Read the model definition and answer for the solid it produces. Units are mm, in the model's axes. A direction names the side the tool comes from. Give positions to 0.01 mm unless a question says otherwise; leave off trailing zeros. Write each loop counter-clockwise with the first axis right and the second up, starting at its lowest first coordinate (ties: lowest second). Pieces come first, ordered by that corner, then holes. Notation, with made-up numbers: (65.5, -40) -> (91.5, -40) arc R26 ccw to (91.5, -5) -> close; hole circle Ø2 at (87.25, 67). An arc over 180 degrees is marked (long way). Write item = value, one per line.
from build123d import *

# Parameters (mm, degrees)
BOSS_EXTRUDE1_DEPTH = 30
SKETCH2_R           = 5
CUT_EXTRUDE1_DEPTH  = 6
SKETCH3_R           = 40
BOSS_EXTRUDE2_DEPTH = 6


with BuildPart() as part:
    # Sketch1 → Boss-Extrude1 (new body)
    with BuildSketch(Plane.XY):
        with BuildLine():
            Line((-2.9, 13.696349879), (-2.9, 16.8))
            Line((-2.9, 16.8), (2.9, 16.8))
            Line((2.9, 16.8), (2.9, 13.696349879))
            ThreePointArc((2.9, 13.696349879), (5.357568053, 12.934313455), (7.634172211, 11.735391542))
            Line((7.634172211, 11.735391542), (9.828784258, 13.930003589))
            Line((9.828784258, 13.930003589), (13.930003589, 9.828784258))
            Line((13.930003589, 9.828784258), (11.735391542, 7.634172211))
            ThreePointArc((11.735391542, 7.634172211), (12.934313455, 5.357568053), (13.696349879, 2.9))
            Line((13.696349879, 2.9), (16.8, 2.9))
            Line((16.8, 2.9), (16.8, -2.9))
            Line((16.8, -2.9), (13.696349879, -2.9))
            ThreePointArc((13.696349879, -2.9), (12.934313455, -5.357568053), (11.735391542, -7.634172211))
            Line((11.735391542, -7.634172211), (13.930003589, -9.828784258))
            Line((13.930003589, -9.828784258), (9.828784258, -13.930003589))
            Line((9.828784258, -13.930003589), (7.634172211, -11.735391542))
            ThreePointArc((7.634172211, -11.735391542), (5.357568053, -12.934313455), (2.9, -13.696349879))
            Line((2.9, -13.696349879), (2.9, -16.8))
            Line((2.9, -16.8), (-2.9, -16.8))
            Line((-2.9, -16.8), (-2.9, -13.696349879))
            ThreePointArc((-2.9, -13.696349879), (-5.357568053, -12.934313455), (-7.634172211, -11.735391542))
            Line((-7.634172211, -11.735391542), (-9.828784258, -13.930003589))
            Line((-9.828784258, -13.930003589), (-13.930003589, -9.828784258))
            Line((-13.930003589, -9.828784258), (-11.735391542, -7.634172211))
            ThreePointArc((-11.735391542, -7.634172211), (-12.934313455, -5.357568053), (-13.696349879, -2.9))
            Line((-13.696349879, -2.9), (-16.8, -2.9))
            Line((-16.8, -2.9), (-16.8, 2.9))
            Line((-16.8, 2.9), (-13.696349879, 2.9))
            ThreePointArc((-13.696349879, 2.9), (-12.934313455, 5.357568053), (-11.735391542, 7.634172211))
            Line((-11.735391542, 7.634172211), (-13.930003589, 9.828784258))
            Line((-13.930003589, 9.828784258), (-9.828784258, 13.930003589))
            Line((-9.828784258, 13.930003589), (-7.634172211, 11.735391542))
            ThreePointArc((-7.634172211, 11.735391542), (-5.357568053, 12.934313455), (-2.9, 13.696349879))
        make_face()
    extrude(amount=BOSS_EXTRUDE1_DEPTH)

    # Sketch2 → Cut-Extrude1 (cut)
    with BuildSketch(Plane(origin=(0, 0, 0), x_dir=(-1, 0, 0), z_dir=(0, 0, -1))):
        Circle(SKETCH2_R)
    extrude(amount=-CUT_EXTRUDE1_DEPTH, mode=Mode.SUBTRACT)

    # Sketch3 → Boss-Extrude2 (add)
    with BuildSketch(Plane.XY.offset(30)):
        Circle(SKETCH3_R)
    extrude(amount=BOSS_EXTRUDE2_DEPTH)


solid = part.part
(1) The part is cut by section B-B on y = 0. Determine the outline of the cut face in (x, z), plus the area to 3 significant figures.
Checks:
outline = (-40, 30) -> (-16.8, 30) -> (-16.8, 0) -> (-5, 0) -> (-5, 6) -> (5, 6) -> (5, 0) -> (16.8, 0) -> (16.8, 30) -> (40, 30) -> (40, 36) -> (-40, 36) -> close
area = 1,430 mm²
(2) A tool of negligible diameter and unlimited length cuts with its end or side. For faces 1 (the cylindrical face through (-5.39, 12.92, 14.79)), 2 (the flat face through (8.7, -12.8, 14.8)), 3 (the flat face through (-12.8, 8.7, 14.8)), 4 (the flat face through (12.8, 8.7, 14.8)), from which of +Z, -Z, +X, -X, +Y, -Y can it reach the whole face along a straight path? Write none if from no direction.
Checks:
face_1 = -Z, +Y
face_2 = -Z, -Y
face_3 = -Z, -X
face_4 = -Z, +X
(3) Consider L1, parallel to Y at x = 0, z = 4.2; L2, parallel to Z at x = -10, y = -16; L3, parallel to X at y = -16, z = 21.5. Determine where each line is inside the solid, lowest interval first.
Checks:
L1 = -16.8 to -5, 5 to 16.8
L2 = 30 to 36
L3 = -2.9 to 2.9
(4) The part is cut by section D-D on y = -15. Determine the outline of the cut face in (x, z), plus the area to 3 significant figures.
Checks:
outline = (-37.08, 30) -> (-2.9, 30) -> (-2.9, 0) -> (2.9, 0) -> (2.9, 30) -> (37.08, 30) -> (37.08, 36) -> (-37.08, 36) -> close
area = 619 mm²
(5) Given P1, Ø2.5, axis at x = 16, z = 15.5, coming from the +Y side; P2, Ø0.9, axis at y = 16, z = 15.5, coming from the -X side; P3, Ø3, axis at y = -0.5, z = 13.5, coming from the +X side; P4, Ø1, axis at x = 18, z = 20, coming from the -Y side, each flat-ended and moving along its own axis, determine where each tip first touches the part or whether it passes through.
Checks:
P1 = 2.9
P2 = -2.9
P3 = 16.8
P4 = through
